from build123d import *

# Parameters (mm, degrees)
F0_R     = 1.5
F1_DEPTH = 6.5


with BuildPart() as f1:
    # F0 (on Front) → F1 (new body)
    with BuildSketch(Plane.XZ):
        Polygon((-8.340434, 4.938039), (-8.340434, -5.261961), (11.659566, -5.261961), (11.659566, 4.238039), (1.659566, 4.238039), (1.045704, 4.938039), (-4.366579, 4.938039), (-5.340434, 4.938039), align=None)
        with Locations((-3.340434, -2.461961)):
            Circle(F0_R, mode=Mode.SUBTRACT)
        with Locations((6.659566, -2.461961)):
            Circle(F0_R, mode=Mode.SUBTRACT)
        with BuildLine():
            Line((-5.340434, 5.956738), (-5.340434, 4.938039))
            Line((-5.340434, 4.938039), (-4.366579, 4.938039))
            Line((-4.366579, 4.938039), (-4.366579, 5.524251))
            Line((-4.366579, 5.524251), (13.146718, 8.761675))
            Line((13.146718, 8.761675), (12.885723, 10.173564))
            ThreePointArc((12.885723, 10.173564), (10.366926, 14.08902), (9.556615, 9.504423))
            Line((9.556615, 9.504423), (9.69852, 8.736767))
            Line((9.69852, 8.736767), (-5.340434, 5.956738))
        make_face()
    extrude(amount=F1_DEPTH)


solid = f1.part
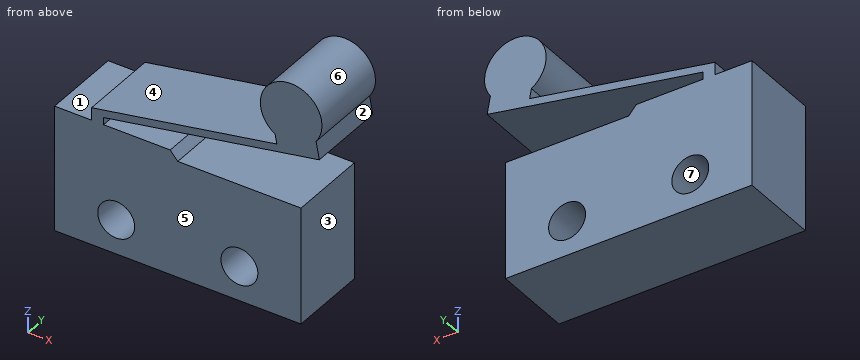
Can you work these out from the model? Positions are in its coordinate system, mm. Face numbers are marked on the shaded views. A direction names the side the tool comes from. Coordinates: 2 decimals unless noted, no trailing zeros. Write each loop counter-clockwise with the first axis right and the second up, starting at its lowest first coordinate (ties: lowest second). Pieces come first, ordered by that corner, then holes. Notation, with made-up numbers: (23, 81) -> (58, 81) arc R22 cw to (58, 106) -> close; hole circle Ø2 at (-10.5, -28). An arc over 180 degrees is marked (long way). Write item = value, one per line.
(1) For pin 1 (3 mm diameter, centred on x = 6.5, y = -3, fed in from +Z); pin 2 (2 mm diameter, centred on y = -4, z = 0, fed in from +X); pin 3 (3 mm diameter, centred on x = 10, y = -5.5, fed in from +Z); pin 4 (1.5 mm diameter, centred on x = -7, y = -2, fed in from +Z), each with a flat end and sliding along its axis, tell me the tip position at first contact or that it passes through.
Verdict:
pin_1 = 8.42
pin_2 = 11.66
pin_3 = 14.14
pin_4 = 4.94
(2) On a 3-axis mill with a long thin cutter (end or side, diameter ignored), from which of +Z, -Z, +X, -X, +Y, -Y can I reach the whole of each face in a straight line? I mean the marked faces 1, 2 and 3. Say none if no direction works.
Verdict:
face_1 = +Z, -X, +Y, -Y
face_2 = +X, +Y, -Y
face_3 = -Z, +X, +Y, -Y
(3) If I drill on probe 1 along Z at (x, y) = (7.5, -0.75); probe 2 along Z at (x, y) = (-3.5, -3.75); probe 3 along X at (y, z) = (-0.25, 0.75), over which ranges is the centre line in solid material (lowest first)?
Verdict:
probe_1 = -5.26 to -3.7, -1.22 to 4.24, 7.72 to 8.33
probe_2 = -5.26 to -3.95, -0.97 to 4.94, 5.68 to 6.3
probe_3 = -8.34 to 11.66
(4) Imagine slicing it at A-A (z = -1.25). Please give me the cut outline in (x, y), and give its area (3 significant figures).
Verdict:
outline = (-8.34, -6.5) -> (-4.22, -6.5) -> (-4.22, 0) -> (-8.34, 0) -> close; (-2.46, -6.5) -> (5.78, -6.5) -> (5.78, 0) -> (-2.46, 0) -> close; (7.54, -6.5) -> (11.66, -6.5) -> (11.66, 0) -> (7.54, 0) -> close
area = 107 mm^2
(5) Imagine slicing it at B-B (x = -4). Please give me the cut outline in (y, z).
Verdict:
outline = (-6.5, -5.26) -> (0, -5.26) -> (0, -3.81) -> (-6.5, -3.81) -> close; (-6.5, -1.11) -> (0, -1.11) -> (0, 4.94) -> (-6.5, 4.94) -> close; (-6.5, 5.59) -> (0, 5.59) -> (0, 6.2) -> (-6.5, 6.2) -> close
(6) Imagine slicing it at D-D (y = -5). Please give me the cut outline in (x, z).
Verdict:
outline = (-8.34, -5.26) -> (11.66, -5.26) -> (11.66, 4.24) -> (1.66, 4.24) -> (1.05, 4.94) -> (-4.37, 4.94) -> (-4.37, 5.52) -> (13.15, 8.76) -> (12.89, 10.17) arc R2.5 ccw (long way) to (9.56, 9.5) -> (9.7, 8.74) -> (-5.34, 5.96) -> (-5.34, 4.94) -> (-8.34, 4.94) -> close; hole circle Ø3 at (-3.34, -2.46); hole circle Ø3 at (6.66, -2.46)
(7) Imagine slicing it at C-C (x = 10). Please give me the cut outline in (y, z), and give its area (3 significant figures).
Verdict:
outline = (-6.5, -5.26) -> (0, -5.26) -> (0, 4.24) -> (-6.5, 4.24) -> close; (-6.5, 8.18) -> (0, 8.18) -> (0, 13.99) -> (-6.5, 13.99) -> close
area = 99.5 mm^2
(8) Thinking about a two-plate mould opening in X: for the marked faces 4, 5, 6 and 7, which applies, +X half, -X half, draft (parallel to the pull), parting line (faces both ways), or undercut?
Verdict:
face_4 = -X half
face_5 = draft
face_6 = parting line
face_7 = undercut
